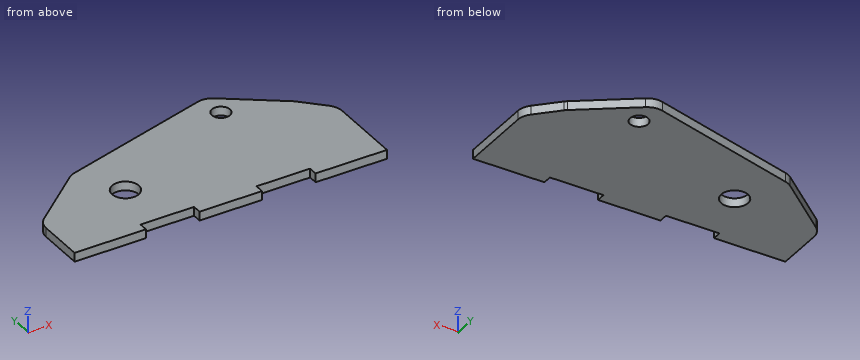
from build123d import *

# Parameters (mm, degrees)
ESQUISSE1_R        = 15
ESQUISSE1_R_2      = 10.125
BOSS_EXTRU_1_DEPTH = 10
CONG_1_R           = 20


with BuildPart() as part:
    # Esquisse1 → Boss.-Extru.1 (new body)
    with BuildSketch(Plane.XY):
        Polygon((350, 0), (350, 90), (320, 120), (250, 170), (70, 120), (0, 61.263025818), (0, 0), (80, 0), (80, 10), (140, 10), (140, 0), (210, 0), (210, 10), (270, 10), (270, 0), align=None)
        with Locations((100, 70)):
            Circle(ESQUISSE1_R, mode=Mode.SUBTRACT)
        with Locations((250, 140)):
            Circle(ESQUISSE1_R_2, mode=Mode.SUBTRACT)
    extrude(amount=BOSS_EXTRU_1_DEPTH)

    # Congé1
    cong_1_edges = [part.edges().sort_by_distance(p)[0] for p in [
        (0, 61.263025818, 5),
        (70, 120, 5),
        (250, 170, 5),
        (320, 120, 5),
        (350, 90, 5),
    ]]
    fillet(cong_1_edges, radius=CONG_1_R)


solid = part.part
Input: part model. Units: mm. Frame: model coordinates. Coordinates: 2 decimals unless noted, no trailing zeros. Loops run counter-clockwise (first coordinate to the right, second up) from the corner with the lowest first, then second, coordinate; pieces in that order, holes last. Notation, with made-up numbers: (-17, -9) - (1, -9) arc R25 cw to (1, 14) - close; hole circle Ø10 at (29, 68). An arc over 180 degrees is marked (long way). Answer in a Markdown table with one row per item. Add a question column.
Item 1: Section query B-B on x = 100. Return the cut outline in (y, z).
Item 2: Section query C-C on z = 7.75. Return the cut outline in (x, y) (3 decimals), then the cut area to 3 significant figures.
Item 3: Line query: line 1 along Y through (x, z) = (250, 8) (3 decimals); line 2 along X through (y, z) = (109, 9.25); line 3 along Y through (x, z) = (306, 1.25). Output: solid intervals per line, ascending. Write a range as [from, to].
Item 4: Contact query for flat-ended pins moving along their axis: P1, Ø3, axis at x = 297, z = 4.5, coming from the +Y side; P2, Ø5, axis at y = 100.5, z = 5.5, coming from the -X side; P3, Ø5, axis at x = 254, z = 6.5, coming from the -Y side; P4, Ø12, axis at x = 250, y = 140, coming from the +Z side. Output: stop coordinate, or through.
Item 5: Section query D-D on x = 177. Return the cut outline in (y, z).
Item 6: Section query A-A on y = 140. Return the cut outline in (x, z) (3 decimals), then the cut area to 3 significant figures.
Recorded:
| question | item | result |
|---|---|---|
| 1 | outline | (10, 0) - (55, 0) - (55, 10) - (10, 10) - close; (85, 0) - (128.33, 0) - (128.33, 10) - (85, 10) - close |
| 2 | outline | (0, 0) - (80, 0) - (80, 10) - (140, 10) - (140, 0) - (210, 0) - (210, 10) - (270, 10) - (270, 0) - (350, 0) - (350, 81.716) arc R20 ccw to (344.142, 95.858) - (321.17, 118.83) arc R20 ccw to (318.653, 120.962) - (257.773, 164.448) arc R20 ccw to (240.796, 167.443) - (74.18, 121.161) arc R20 ccw to (66.677, 117.212) - (7.144, 67.258) arc R20 ccw to (0, 51.937) - close; hole circle Ø30 at (100, 70); hole circle Ø20.25 at (250, 140) |
| 2 | area | 43,500 mm^2 |
| 3 | line 1 | [10, 129.875], [150.125, 167.799] |
| 3 | line 2 | [56.89, 331] |
| 3 | line 3 | [0, 130] |
| 4 | P1 | y = 137.5 |
| 4 | P2 | x = 43.78 |
| 4 | P3 | y = 10 |
| 4 | P4 | through |
| 5 | outline | (0, 0) - (149.72, 0) - (149.72, 10) - (0, 10) - close |
| 6 | outline | (142, 0) - (239.875, 0) - (239.875, 10) - (142, 10) - close; (260.125, 0) - (292, 0) - (292, 10) - (260.125, 10) - close |
| 6 | area | 1,300 mm^2 |
